The drawing under review shows one solid part. Ordinate dimensions are in mm from its lowest x, y, z. A direction names the side the tool comes from. Coordinates: 2 decimals unless noted, no trailing zeros. Write each loop counter-clockwise with the first axis right and the second up, starting at its lowest first coordinate (ties: lowest second). Pieces come first, ordered by that corner, then holes. Notation, with made-up numbers: (-23.75, 20.5) - (31.25, 20.5) arc R20 ccw to (31.25, 47.5) - close; hole circle Ø8 at (-4, -4.75). An arc over 180 degrees is marked (long way). Put each result on its own line as item: value. Start each with the question number.
Item 1: Consider section C-C on x = 56. Give the boundary of the cut face in (y, z), then the cut area to 3 significant figures.
Item 2: To check wall thickness, follow L1, parallel to X at y = 4.5, z = 14.5; L2, parallel to Z at x = 12, y = 13; L3, parallel to X at y = 21, z = 24.25. State the ranges of each line that lie inside material, in increasing order. Write a range as [from, to].
Item 3: Consider section A-A on z = 13.4. Give the boundary of the cut face in (x, y).
Item 4: Consider section D-D on z = 2.5. Give the boundary of the cut face in (x, y), then the cut area to 3 significant figures.
Item 5: Machinability: for the marked faces 1, 2 and 3, which of the approach directions +Z, -Z, +X, -X, +Y, -Y give a long, thin tool a straight path to every point of the face, cutting with its end or side? Answer none if there is none.
Item 6: Consider section B-B on y = 13.4. Give the boundary of the cut face in (x, z).
Item 7: For pin 1 (1.5 mm diameter, centred on y = 23.5, z = 6.5, fed in from -X); pin 2 (5 mm diameter, centred on x = 24.5, y = 17.5, fed in from +Z); pin 3 (1.5 mm diameter, centred on y = 12, z = 24, fed in from +X); pin 4 (13.5 mm diameter, centred on y = 13.5, z = 7.5, fed in from +X), all flat-tipped, find the tip position at first contact; note any pin that passes through.
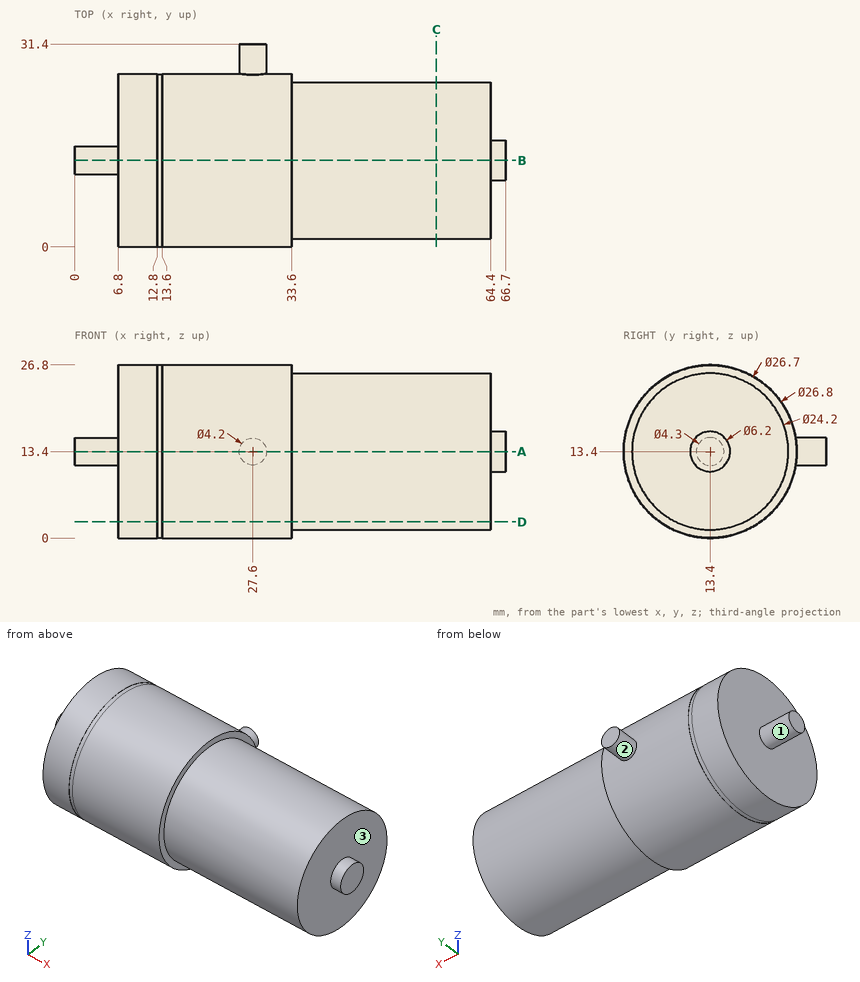
Report:
1. outline: circle Ø24.2 at (13.4, 13.4)
1. area: 460 mm²
2. L1: [6.8, 64.4]
2. L2: [0.01, 26.79]
2. L3: [6.8, 33.6]
3. outline: (0, 11.25) - (6.8, 11.25) - (6.8, 0) - (12.8, 0) - (12.8, 0.05) - (13.6, 0.05) - (13.6, 0) - (33.6, 0) - (33.6, 1.3) - (64.4, 1.3) - (64.4, 10.3) - (66.7, 10.3) - (66.7, 16.5) - (64.4, 16.5) - (64.4, 25.5) - (33.6, 25.5) - (33.6, 26.8) - (29.7, 26.8) - (29.7, 31.4) - (25.5, 31.4) - (25.5, 26.8) - (13.6, 26.8) - (13.6, 26.75) - (12.8, 26.75) - (12.8, 26.8) - (6.8, 26.8) - (6.8, 15.55) - (0, 15.55) - close
4. outline: (6.8, 5.61) - (12.8, 5.61) - (12.8, 5.69) - (13.6, 5.69) - (13.6, 5.61) - (33.6, 5.61) - (33.6, 8.15) - (64.4, 8.15) - (64.4, 18.65) - (33.6, 18.65) - (33.6, 21.19) - (13.6, 21.19) - (13.6, 21.11) - (12.8, 21.11) - (12.8, 21.19) - (6.8, 21.19) - close
4. area: 741 mm²
5. face 1: -X
5. face 2: +Y
5. face 3: +X
6. outline: (0, 11.25) - (6.8, 11.25) - (6.8, 0) - (12.8, 0) - (12.8, 0.05) - (13.6, 0.05) - (13.6, 0) - (33.6, 0) - (33.6, 1.3) - (64.4, 1.3) - (64.4, 10.3) - (66.7, 10.3) - (66.7, 16.5) - (64.4, 16.5) - (64.4, 25.5) - (33.6, 25.5) - (33.6, 26.8) - (13.6, 26.8) - (13.6, 26.75) - (12.8, 26.75) - (12.8, 26.8) - (6.8, 26.8) - (6.8, 15.55) - (0, 15.55) - close
7. pin 1: x = 6.8
7. pin 2: z = 26.7
7. pin 3: x = 64.4
7. pin 4: x = 66.7
